Build history of the part. All positions in model axes, mm. A direction names the side the tool comes from. Round coordinates to 2 decimals unless told otherwise and drop trailing zeros. Write each loop counter-clockwise with the first axis right and the second up, starting at its lowest first coordinate (ties: lowest second). Pieces come first, ordered by that corner, then holes.
Item 1: Mould opens along Z. For faces 1 (the cylindrical face through (-1.283, 22.219, 6.195)), 2 (the cylindrical face through (9.5, 19.9, 0.8)), 3 (the flat face through (0, 28.1, 3)) say: +Z half, -Z half, draft (parallel to the pull), parting line (faces both ways), or undercut.
Item 2: 3-axis set-ups, long thin cutter, end or side, ignore diameter. For faces 4 (the cylindrical face through (-9.5, 19.9, 0.8)), 5 (the flat face through (0, 0, -9)), 6 (the flat face through (6, 23.32, 1)), 7 (the flat face through (0, 20, -0.25)): which of +Z, -Z, +X, -X, +Y, -Y reach the whole face in a straight line?
Item 3: Band-saw the part on A-A, the plane y = 5.5. Write the cut outline in (x, z).
Item 4: Drop flat-ended pins along their axis: pin 1 Ø10 at (x, z) = (-25, 12) entering from +Y; pin 2 Ø8 at (x, z) = (1.5, 23.5) entering from +Y; pin 3 Ø3.5 at (x, y) = (2, 20.5) entering from -Z. Give the stop position or say it passes through.
Item 5: Wall check: probe 1 along Y at (x, z) = (9, 12.5); probe 2 along X at (y, z) = (-26.5, 20.5); probe 3 along X at (y, z) = (-13, 14.5). Give the ranges that are in metal, low to high.
```python
from build123d import *

# Parameters (mm, degrees)
SKETCH2_R                       = 3.35
BOSS_EXTRUDE1_DEPTH             = 11.6
BOSS_EXTRUDE2_DEPTH             = 6.82
SKETCH8_R                       = 7.5
BOSS_EXTRUDE3_DEPTH             = 80
BOSS_EXTRUDE3_DIRECTION_2_REACH = 50.394


with BuildPart() as part:
    # Sketch1 → Revolve1 (revolve)
    with BuildSketch(Plane(origin=(0, 0, 0), x_dir=(0, 0, -1), z_dir=(1, 0, 0)), mode=Mode.PRIVATE) as revolve1_sk:
        Polygon((0, 16.5), (0, 0), (20.5, 0), (10.75, 16.5), align=None)
    revolve(revolve1_sk.sketch.rotate(Axis((0, 16.5, 0), (0, -1, 0)), 180), axis=Axis((0, 16.5, 0), (0, -1, 0)))

    # Sketch2 → Boss-Extrude1 (add)
    with BuildSketch(Plane(origin=(0, 16.5, 0), x_dir=(1, 0, 0), z_dir=(0, 1, 0))):
        with Locations(Location((0, -3.1, 0), (0, 0, 270))):
            Circle(SKETCH2_R)
    extrude(amount=BOSS_EXTRUDE1_DEPTH)

    # Sketch3 → Boss-Extrude2 (add)
    with BuildSketch(Plane(origin=(0, 16.5, 0), x_dir=(1, 0, 0), z_dir=(0, 1, 0))):
        with BuildLine():
            Line((-8.425, 0.25), (8.425, 0.25))
            ThreePointArc((8.425, 0.25), (9.5, -0.825), (8.425, -1.9))
            Line((8.425, -1.9), (-8.425, -1.9))
            ThreePointArc((-8.425, -1.9), (-9.5, -0.825), (-8.425, 0.25))
        make_face()
    extrude(amount=BOSS_EXTRUDE2_DEPTH)

    # Sketch8 → Boss-Extrude3 (add)
    with BuildSketch(Plane(origin=(-6.20436158, -4.094388045, 3.839162967), x_dir=(0.5261928654830319, 0, 0.8503652558252577), z_dir=(-0.7415774099490876, -0.4893824517488441, 0.458876629360761))):
        with Locations(Location((0, -1, 0), (0, 0, 286.847482278))):
            Circle(SKETCH8_R)
    extrude(amount=BOSS_EXTRUDE3_DEPTH)

    # Sketch8 → Boss-Extrude3 direction 2 (add, up to next)
    with BuildSketch(Plane(origin=(-6.20436158, -4.094388045, 3.839162967), x_dir=(0.5261928654830319, 0, 0.8503652558252577), z_dir=(-0.7415774099490876, -0.4893824517488441, 0.458876629360761)), mode=Mode.PRIVATE) as boss_extrude3_direction_2_sk1:
        with Locations(Location((0, -1, 0), (0, 0, 286.847482278))):
            Circle(SKETCH8_R)
    boss_extrude3_direction_2_tool1 = extrude(boss_extrude3_direction_2_sk1.sketch, amount=-BOSS_EXTRUDE3_DIRECTION_2_REACH, mode=Mode.PRIVATE) - part.part
    add(boss_extrude3_direction_2_tool1.solids().sort_by_distance((-5.788208, -4.966457, 3.581653))[0])


solid = part.part
```
Results:
1. face 1: undercut
1. face 2: parting line
1. face 3: draft
2. face 4: -X, +Y
2. face 5: none
2. face 6: -Z, +X, +Y
2. face 7: -Z, +X, -X, +Y
3. outline: circle Ø34.5 at (0, 0)
4. pin 1: stops at y = -5.5
4. pin 2: stops at y = 1.61
4. pin 3: stops at z = -0.25
5. probe 1: y = 0 to 8.63
5. probe 2: x = -46.54 to -25.35
5. probe 3: x = -31.08 to -9.97
